The listing builds one solid part. Answer for the finished solid, in the listing's coordinates (mm). A direction names the side the tool comes from. Coordinates: 2 decimals unless noted, no trailing zeros. Write each loop counter-clockwise with the first axis right and the second up, starting at its lowest first coordinate (ties: lowest second). Pieces come first, ordered by that corner, then holes.
(1) For a pull along Y with two mould halves and no side action, classify faces 5 (the flat face through (0, 12.7, 0)), 6 (the flat face through (6.965, 0, 4)), 7 (the flat face through (2, 7.493, 3)) as +Y half, -Y half, draft (parallel to the pull), parting line (faces both ways), or undercut.
(2) The part is cut by section D-D on y = 8.75. Determine the outline of the cut face in (x, z).
(3) The part is cut by section B-B on x = 12.5. Determine the outline of the cut face in (y, z), plus the area to 3 significant figures.
(4) The part is cut by section C-C on z = -4.25. Determine the outline of the cut face in (x, y), plus the area to 3 significant figures.
(5) Which of the six approach directions +Z, -Z, +X, -X, +Y, -Y give full straight-line access (tool end or side, diameter ignored) to faces 1 (the flat face through (15, 5, 2.794)), 2 (the flat face through (-0.698, 10, 3)), 3 (the flat face through (-2.128, 0, 4)), 4 (the flat face through (2, 10, 3.937))?
(6) The part is cut by section A-A on y = -0.75. Determine the outline of the cut face in (x, z) (3 decimals).
(7) Given P1, Ø2.5, axis at y = 0.5, z = 4, coming from the -X side; P2, Ø0.7, axis at y = 10.5, z = -4.5, coming from the +X side; P3, Ø0.7, axis at y = 10.5, z = -3.5, coming from the -X side, each flat-ended and moving along its own axis, determine where each tip first touches the part or whether it passes through.
(8) Straight lines are drawn through the part: line 1 (Y direction, x = -10, z = -4.5); line 2 (Z direction, x = -11.5, y = -8); line 3 (Z direction, x = 2, y = 10). For each, find the intervals that lie inside material, in ascending order.
from build123d import *

# Parameters (mm, degrees)
F0_W     = 40.6
F0_H     = 25.4
F0_W_2   = 0.64
F0_H_2   = 0.64
F0_W_3   = 9.0932
F0_H_3   = 10.7696
F0_W_4   = 7.4422
F0_H_4   = 8.763
F0_W_5   = 6.23316
F0_H_5   = 4.699
F1_DEPTH = 2.667
F2_DEPTH = 5.588
F3_DEPTH = 3.937
F4_DEPTH = 2.794
F5_DEPTH = 2.54
F6_DEPTH = 5.461


with BuildPart() as f1:
    # F0 (on Top) → F1 (new body)
    with BuildSketch(Plane.XY):
        Rectangle(F0_W, F0_H)
        with Locations((-10.14, -2.54)):
            Rectangle(F0_W_2, F0_H_2, mode=Mode.SUBTRACT)
        with Locations((10.18, -10.16)):
            Rectangle(F0_W_2, F0_H_2, mode=Mode.SUBTRACT)
        with Locations((-10.14, 2.54)):
            Rectangle(F0_W_2, F0_H_2, mode=Mode.SUBTRACT)
        with Locations((-10.14, 10.16)):
            Rectangle(F0_W_2, F0_H_2, mode=Mode.SUBTRACT)
        with Locations((2.4184, 0.4572)):
            Rectangle(F0_W_3, F0_H_3, mode=Mode.SUBTRACT)
        with Locations((14.9279, 5.2705)):
            Rectangle(F0_W_4, F0_H_4, mode=Mode.SUBTRACT)
        with Locations((2.4184, 9.8425)):
            Rectangle(F0_W_5, F0_H_5, mode=Mode.SUBTRACT)
        with Locations((10.18, 10.16)):
            Rectangle(F0_W_2, F0_H_2, mode=Mode.SUBTRACT)
        with Locations((-10.14, 10.16)):
            Rectangle(F0_W_2, F0_H_2)
        with Locations((-10.14, 2.54)):
            Rectangle(F0_W_2, F0_H_2)
        with Locations((-10.14, -2.54)):
            Rectangle(F0_W_2, F0_H_2)
        with Locations((10.18, 10.16)):
            Rectangle(F0_W_2, F0_H_2)
        with Locations((10.18, -10.16)):
            Rectangle(F0_W_2, F0_H_2)
    extrude(amount=F1_DEPTH)

    # F0 (on Top) → F2 (join)
    with BuildSketch(Plane.XY):
        with Locations((2.4184, 0.4572)):
            Rectangle(F0_W_3, F0_H_3)
    extrude(amount=F2_DEPTH)

    # F0 (on Top) → F3 (join)
    with BuildSketch(Plane.XY):
        with Locations((2.4184, 9.8425)):
            Rectangle(F0_W_5, F0_H_5)
    extrude(amount=F3_DEPTH)

    # F0 (on Top) → F4 (join)
    with BuildSketch(Plane.XY):
        with Locations((14.9279, 5.2705)):
            Rectangle(F0_W_4, F0_H_4)
    extrude(amount=F4_DEPTH)

    # F0 (on Top) → F5 (join)
    with BuildSketch(Plane.XY):
        Rectangle(F0_W, F0_H)
        with Locations((-10.14, -2.54)):
            Rectangle(F0_W_2, F0_H_2, mode=Mode.SUBTRACT)
        with Locations((10.18, -10.16)):
            Rectangle(F0_W_2, F0_H_2, mode=Mode.SUBTRACT)
        with Locations((-10.14, 2.54)):
            Rectangle(F0_W_2, F0_H_2, mode=Mode.SUBTRACT)
        with Locations((-10.14, 10.16)):
            Rectangle(F0_W_2, F0_H_2, mode=Mode.SUBTRACT)
        with Locations((2.4184, 0.4572)):
            Rectangle(F0_W_3, F0_H_3, mode=Mode.SUBTRACT)
        with Locations((14.9279, 5.2705)):
            Rectangle(F0_W_4, F0_H_4, mode=Mode.SUBTRACT)
        with Locations((2.4184, 9.8425)):
            Rectangle(F0_W_5, F0_H_5, mode=Mode.SUBTRACT)
        with Locations((10.18, 10.16)):
            Rectangle(F0_W_2, F0_H_2, mode=Mode.SUBTRACT)
        with Locations((-10.14, -2.54)):
            Rectangle(F0_W_2, F0_H_2)
        with Locations((-10.14, 2.54)):
            Rectangle(F0_W_2, F0_H_2)
        with Locations((-10.14, 10.16)):
            Rectangle(F0_W_2, F0_H_2)
        with Locations((10.18, 10.16)):
            Rectangle(F0_W_2, F0_H_2)
        with Locations((2.4184, 9.8425)):
            Rectangle(F0_W_5, F0_H_5)
        with Locations((2.4184, 0.4572)):
            Rectangle(F0_W_3, F0_H_3)
        with Locations((14.9279, 5.2705)):
            Rectangle(F0_W_4, F0_H_4)
        with Locations((10.18, -10.16)):
            Rectangle(F0_W_2, F0_H_2)
    extrude(amount=-F5_DEPTH)

    # F0 (on Top) → F6 (join)
    with BuildSketch(Plane.XY):
        with Locations((-10.14, -2.54)):
            Rectangle(F0_W_2, F0_H_2)
        with Locations((-10.14, 2.54)):
            Rectangle(F0_W_2, F0_H_2)
        with Locations((-10.14, 10.16)):
            Rectangle(F0_W_2, F0_H_2)
        with Locations((10.18, 10.16)):
            Rectangle(F0_W_2, F0_H_2)
        with Locations((10.18, -10.16)):
            Rectangle(F0_W_2, F0_H_2)
    extrude(amount=-F6_DEPTH)


solid = f1.part
Model answer:
1. face 5: +Y half
1. face 6: draft
1. face 7: undercut
2. outline: (-20.3, -2.54) - (20.3, -2.54) - (20.3, 2.67) - (18.65, 2.67) - (18.65, 2.79) - (11.21, 2.79) - (11.21, 2.67) - (5.53, 2.67) - (5.53, 3.94) - (-0.7, 3.94) - (-0.7, 2.67) - (-20.3, 2.67) - close
3. outline: (-12.7, -2.54) - (12.7, -2.54) - (12.7, 2.67) - (9.65, 2.67) - (9.65, 2.79) - (0.89, 2.79) - (0.89, 2.67) - (-12.7, 2.67) - close
3. area: 133 mm2
4. outline: (-10.46, -2.86) - (-9.82, -2.86) - (-9.82, -2.22) - (-10.46, -2.22) - close; (-10.46, 2.22) - (-9.82, 2.22) - (-9.82, 2.86) - (-10.46, 2.86) - close; (-10.46, 9.84) - (-9.82, 9.84) - (-9.82, 10.48) - (-10.46, 10.48) - close; (9.86, -10.48) - (10.5, -10.48) - (10.5, -9.84) - (9.86, -9.84) - close; (9.86, 9.84) - (10.5, 9.84) - (10.5, 10.48) - (9.86, 10.48) - close
4. area: 2.05 mm2
5. face 1: +Z, +X, +Y, -Y
5. face 2: +Z, -X, +Y
5. face 3: +Z, -X, +Y, -Y
5. face 4: +Z, +X, -X, +Y
6. outline: (-20.3, -2.54) - (20.3, -2.54) - (20.3, 2.667) - (6.965, 2.667) - (6.965, 5.588) - (-2.128, 5.588) - (-2.128, 2.667) - (-20.3, 2.667) - close
7. P1: stops at x = -2.13
7. P2: stops at x = 10.5
7. P3: stops at x = -10.46
8. line 1: y = -2.86 to -2.22, 2.22 to 2.86, 9.84 to 10.48
8. line 2: z = -2.54 to 2.67
8. line 3: z = -2.54 to 3.94
